Could you check a few things on this model? Use its own coordinates, in mm. A direction names the side the tool comes from. Give positions to 0.01 mm unless a question says otherwise; leave off trailing zeros. Write each loop counter-clockwise with the first axis right and the second up, starting at its lowest first coordinate (ties: lowest second). Pieces come first, ordered by that corner, then holes. Notation, with made-up numbers: (58.5, -19) - (87.5, -19) arc R18 ccw to (87.5, -7) - close; hole circle Ø9 at (-14, -28.75). An arc over 180 degrees is marked (long way). Use one line per item in the form item = value.
```python
from build123d import *

# Parameters (mm, degrees)
F1_DEPTH  = 13.5
F3_DEPTH  = 30
F5_DEPTH  = 3
F7_D      = 10
F8_R      = 7
F9_DEPTH  = 40
F10_R     = 7
F11_DEPTH = 40
F13_DEPTH = 45


with BuildPart() as f1:
    # F0 (on Front) → F1 (new body, symmetric)
    with BuildSketch(Plane.XZ):
        with BuildLine():
            add(Edge.make_bspline(
                [(-41.5, 0), (-40.6509190798, 35.0818894804), (0.6570294499, 61.9181105196), (39.3368601799, 35.0818894804), (41.5, 0)],
                knots=[0, 0, 0, 0, 0.5, 1, 1, 1, 1], degree=3))
            ThreePointArc((-41.5, 0), (0, -41.5), (41.5, 0))
        make_face()
    extrude(amount=F1_DEPTH, both=True)

    # F2 (on face) → F3 (cut)
    with BuildSketch(Plane.XZ.offset(13.5)):
        with BuildLine():
            ThreePointArc((32.5374414571, -12.8963135596), (34.3788485191, -6.5646610347), (35, 0))
            ThreePointArc((35, 0), (26.6213074089, 22.7223676548), (5.4968004663, 34.5656648227))
            ThreePointArc((5.4968004663, 34.5656648227), (6.7399251447, 32.4431879402), (7.1720870792, 30.021720793))
            ThreePointArc((7.1720870792, 30.021720793), (-2.286987081, 23.4678704533), (-5.1001855708, 34.6264076558))
            ThreePointArc((-5.1001855708, 34.6264076558), (-30.0956422284, 17.8676332753), (-32.8417131072, -12.1004909067))
            ThreePointArc((-32.8417131072, -12.1004909067), (-25.0470149854, -7.6099732464), (-19.2668672949, -14.5028652623))
            ThreePointArc((-19.2668672949, -14.5028652623), (-21.8672756585, -19.947458308), (-27.7364654185, -21.3468612702))
            ThreePointArc((-27.7364654185, -21.3468612702), (-0.4437125722, -34.9971873035), (27.186343602, -22.0432012547))
            ThreePointArc((27.186343602, -22.0432012547), (19.8715130661, -11.6252013242), (32.5374414571, -12.8963135596))
        make_face()
    extrude(amount=-F3_DEPTH, mode=Mode.SUBTRACT)

    # F4 (on face) → F5 (cut)
    with BuildSketch(Plane.XZ.offset(13.5)):
        with BuildLine():
            add(Edge.make_bspline(
                [(-41.5, 0), (-40.6509190798, 35.0818894804), (0.6570294499, 61.9181105196), (39.3368601799, 35.0818894804), (41.5, 0)],
                knots=[0, 0, 0, 0, 0.5, 1, 1, 1, 1], degree=3))
            ThreePointArc((-41.5, 0), (0, -41.5), (41.5, 0))
        make_face()
        with BuildLine():
            ThreePointArc((-5.5944102498, 33.9900338545), (0.2188459884, 34.4261095338), (6.02153387, 33.8667139323))
            ThreePointArc((6.02153387, 33.8667139323), (5.7700864546, 34.2243869697), (5.4968004663, 34.5656648227))
            ThreePointArc((5.4968004663, 34.5656648227), (30.4107010386, 17.3259707474), (32.5374414571, -12.8963135596))
            ThreePointArc((32.5374414571, -12.8963135596), (32.2505420404, -12.1862967222), (31.8878008438, -11.5118680686))
            ThreePointArc((31.8878008438, -11.5118680686), (29.2191511765, -17.1200357859), (25.5785678665, -22.1518733584))
            ThreePointArc((25.5785678665, -22.1518733584), (26.3855932866, -22.1439565844), (27.186343602, -22.0432012547))
            ThreePointArc((27.186343602, -22.0432012547), (-0.4437125722, -34.9971873035), (-27.7364654185, -21.3468612702))
            ThreePointArc((-27.7364654185, -21.3468612702), (-27.0814923312, -21.4553026803), (-26.4191917867, -21.5012077267))
            ThreePointArc((-26.4191917867, -21.5012077267), (-29.8477517846, -16.5307845373), (-32.3469371921, -11.0340398062))
            ThreePointArc((-32.3469371921, -11.0340398062), (-32.6167533089, -11.5568598976), (-32.8417131072, -12.1004909067))
            ThreePointArc((-32.8417131072, -12.1004909067), (-30.0956422284, 17.8676332753), (-5.1001855708, 34.6264076558))
            ThreePointArc((-5.1001855708, 34.6264076558), (-5.3564618775, 34.3153377337), (-5.5944102498, 33.9900338545))
        make_face(mode=Mode.SUBTRACT)
    extrude(amount=-F5_DEPTH, mode=Mode.SUBTRACT)

    # F7 (through all)
    with Locations(Plane(origin=(0, 13.5, 0), x_dir=(-1, 0, 0), z_dir=(0, 1, 0))):
        with Locations((0.0923887911, 30.0220718413), (-26.0460712844, -14.9310248805), (25.9536824933, -15.0910469608)):
            Hole(F7_D / 2)

    # F8 (on Top) → F9 (cut)
    with BuildSketch(Plane.XY):
        with Locations((0, 13.2217486843)):
            Circle(F8_R)
    extrude(amount=-F9_DEPTH, mode=Mode.SUBTRACT)

    # F10 (on Right) → F11 (cut, symmetric)
    with BuildSketch(Plane.YZ):
        with Locations((13.1687597471, 0)):
            Circle(F10_R)
    extrude(amount=F11_DEPTH, both=True, mode=Mode.SUBTRACT)

    # F12 (on Front) → F13 (cut, symmetric)
    with BuildSketch(Plane.XZ):
        with BuildLine():
            add(Edge.make_bspline(
                [(-37.1117404138, 12.9166683182), (-31.8909446924, 33.2991668752), (-20.4388675878, 42.310272007), (-7.7872653969, 44.7230026175)],
                knots=[0, 0, 0, 0, 0.415839322, 0.415839322, 0.415839322, 0.415839322], degree=3))
            ThreePointArc((-37.1117404138, 12.9166683182), (-39.1537586618, 3.332383477), (-38.7608190529, -6.4591410676))
            Line((-38.7608190529, -6.4591410676), (-17.4803026021, -6.4591410676))
            Line((-17.4803026021, -6.4591410676), (-17.4803026021, -23.350475356))
            Line((-17.4803026021, -23.350475356), (-31.6050138053, -23.350475356))
            ThreePointArc((-31.6050138053, -23.350475356), (-0.2633451611, -39.2944302199), (31.2892064192, -23.77198264))
            Line((31.2892064192, -23.77198264), (17.6453739405, -23.77198264))
            Line((17.6453739405, -23.77198264), (17.6453739405, -6.6884830925))
            Line((17.6453739405, -6.6884830925), (38.7219032449, -6.6884830925))
            ThreePointArc((38.7219032449, -6.6884830925), (39.1634506664, 3.2164777144), (37.1117404138, 12.9166683182))
            add(Edge.make_bspline(
                [(8.172452372, 44.5784830349), (20.7986586816, 41.9557269194), (32.3701441874, 32.8654666183), (37.1117404138, 12.9166683182)],
                knots=[0.5879451924, 0.5879451924, 0.5879451924, 0.5879451924, 1, 1, 1, 1], degree=3))
            Line((8.172452372, 44.5784830349), (8.172452372, 21.7333426662))
            Line((8.172452372, 21.7333426662), (-7.7872653969, 21.7333426662))
            Line((-7.7872653969, 21.7333426662), (-7.7872653969, 44.7230026175))
        make_face()
    extrude(amount=F13_DEPTH, both=True, mode=Mode.SUBTRACT)


solid = f1.part
```
1. If I drill on line 1 (X direction, y = 11.25, z = 32); line 2 (Z direction, x = 4.5, y = -1.75); line 3 (Z direction, x = 3, y = 2), over which ranges is the centre line in solid material (lowest first)? Write a range as from..to.
Response values:
line_1 = -32.44..-28.35, -6.54..-4.68, 4.5..6.89, 28.45..31.87
line_2 = -41.26..-39.04, 24.52..28.04, 32..48.27
line_3 = -41.39..-39.18, 23.62..26.09, 33.95..48.4
2. Imagine slicing it at B-B, the plane x = 0. State how many separate pieces and enclosed holes the cut face has, and give its area (3 significant figures).
Response values:
separate_pieces = 3
enclosed_holes = 0
area = 425 mm²
3. Imagine slicing it at A-A, the plane z = -28. List the corners of the cut face in (x, y) for me.
Response values:
outline = (-30.63, -10.5) - (-27.57, -10.5) - (-27.57, 13.5) - (-30.63, 13.5) - close; (27.57, -10.5) - (30.63, -10.5) - (30.63, 13.5) - (27.57, 13.5) - close
4. Which directions (+Z, -Z, +X, -X, +Y, -Y) give clear straight access to the entire face, cutting with the end or side of a thin tool? Please do faces 1 (the face through (-37, 0, -6.459)), 2 (the face through (-0.91, 1.33, -41.49)).
Response values:
face_1 = +Y, -Y
face_2 = -Z, +Y, -Y
5. If we mould it in two halves opening along Z, with no side actions, what happens to faces 3 (the face through (-40, 11, 0)), 4 (the face through (31.436, -12.021, -12.672)), 5 (the face through (-24, -13.5, -10))? For each: pulls with the +Z half, pulls with the -Z half, needs draft (parallel to the pull), parting line crosses it, or undercut.
Response values:
face_3 = undercut
face_4 = pulls with the -Z half
face_5 = needs draft
6. For pin 1 (10 mm diameter, centred on x = -20, z = -4, fed in from -Y); pin 2 (5 mm diameter, centred on x = 37, y = -4.5, fed in from +Z); pin 3 (6 mm diameter, centred on x = -25.5, y = -5.5, fed in from -Z); pin 4 (8.5 mm diameter, centred on y = 0.5, z = 42, fed in from -X), each with a flat end and sliding along its axis, tell me the tip position at first contact or that it passes through.
Response values:
pin_1 = through
pin_2 = 27.65
pin_3 = -34.87
pin_4 = -27.58
